Input: part model. Units: mm. Frame: model coordinates. A direction names the side the tool comes from. Give positions to 0.01 mm unless a question says otherwise; leave off trailing zeros. Loops run counter-clockwise (first coordinate to the right, second up) from the corner with the lowest first, then second, coordinate; pieces in that order, holes last. Notation, with made-up numbers: (-20, -5) -> (34, -5) arc R10 ccw to (34, 9) -> close; hole circle Ø7 at (-4.5, 84.25). An arc over 180 degrees is marked (long way). Answer as a JSON object with one key per item and string values.
```python
from build123d import *

# Parameters (mm, degrees)
BOSS_EXTRUDE2_OUTLINE_R   = 1.35
BOSS_EXTRUDE2_OUTLINE_W   = 11
BOSS_EXTRUDE2_OUTLINE_H   = 69
BOSS_EXTRUDE2_OUTLINE_R_2 = 12.095
BOSS_EXTRUDE2_OUTLINE_R_3 = 1.143
BOSS_EXTRUDE2_DEPTH       = 3.175
CUT_EXTRUDE1_DEPTH        = 6.35
FILLET1_R                 = 0.5


# Read off the part's stored shape, not the designer's step: Boss-Extrude2
with BuildPart() as part:
    # Boss-Extrude2 outline → Boss-Extrude2 (new body)
    with BuildSketch(Plane(origin=(0, 0, 0), x_dir=(1, 0, 0), z_dir=(0, 1, 0))):
        with BuildLine():
            ThreePointArc((-13.319120077, -43.925216134), (-10.126305957, -47.701325441), (-5.276948898, -48.669209533))
            ThreePointArc((-5.276948898, -48.669209533), (0, -48.302004425), (5.276948898, -48.669209533))
            ThreePointArc((5.276948898, -48.669209533), (10.126305957, -47.701325441), (13.319120077, -43.925216134))
            Line((13.319120077, -43.925216134), (17.904063474, -31.950549264))
            Line((17.904063474, -31.950549264), (23.040433069, -33.917198033))
            Line((23.040433069, -33.917198033), (18.455489673, -45.891864903))
            ThreePointArc((18.455489673, -45.891864903), (18.309924074, -50.834725832), (21.272807595, -54.79381471))
            ThreePointArc((21.272807595, -54.79381471), (26.466137741, -58.99482374), (30.845959646, -64.038266509))
            ThreePointArc((30.845959646, -64.038266509), (30.722917613, -61.793165345), (29.939937248, -59.685427143))
            Line((29.939937248, -59.685427143), (23.761921217, -48.539993511))
            Line((23.761921217, -48.539993511), (28.572329606, -45.873540599))
            Line((28.572329606, -45.873540599), (34.750345491, -57.018976288))
            ThreePointArc((34.750345491, -57.018976288), (39.797694407, -60.728851606), (45.899993549, -59.314337155))
            ThreePointArc((45.899993549, -59.314337155), (49.682691748, -56.183895741), (53.252452412, -52.812652955))
            ThreePointArc((53.252452412, -52.812652955), (55.400241506, -46.895968251), (52.284336639, -41.426846498))
            Line((52.284336639, -41.426846498), (41.919203487, -33.87844485))
            Line((41.919203487, -33.87844485), (45.152040904, -29.428864843))
            Line((45.152040904, -29.428864843), (55.532494673, -36.970706015))
            ThreePointArc((55.532494673, -36.970706015), (61.693781059, -38.244294688), (66.657056834, -34.377852961))
            ThreePointArc((66.657056834, -34.377852961), (74.442262703, 9.129596032), (56.374397975, 49.466425512))
            ThreePointArc((56.374397975, 49.466425512), (50.654117331, 52.01932544), (44.991624855, 49.340690033))
            Line((44.991624855, 49.340690033), (36.78429665, 39.55957716))
            Line((36.78429665, 39.55957716), (32.571052213, 43.094909013))
            Line((32.571052213, 43.094909013), (40.778380417, 52.876021886))
            ThreePointArc((40.778380417, 52.876021886), (42.433039833, 58.917628535), (38.925607882, 64.107698843))
            ThreePointArc((38.925607882, 64.107698843), (0, 75), (-38.925607882, 64.107698843))
            ThreePointArc((-38.925607882, 64.107698843), (-42.433039833, 58.917628535), (-40.778380417, 52.876021886))
            Line((-40.778380417, 52.876021886), (-32.571052213, 43.094909013))
            Line((-32.571052213, 43.094909013), (-36.78429665, 39.55957716))
            Line((-36.78429665, 39.55957716), (-44.991624855, 49.340690033))
            ThreePointArc((-44.991624855, 49.340690033), (-50.654117331, 52.01932544), (-56.374397975, 49.466425512))
            ThreePointArc((-56.374397975, 49.466425512), (-74.442262703, 9.129596032), (-66.657056834, -34.377852961))
            ThreePointArc((-66.657056834, -34.377852961), (-61.693781059, -38.244294688), (-55.532494673, -36.970706015))
            Line((-55.532494673, -36.970706015), (-45.152040904, -29.428864843))
            Line((-45.152040904, -29.428864843), (-41.919203487, -33.87844485))
            Line((-41.919203487, -33.87844485), (-52.284336639, -41.426846498))
            ThreePointArc((-52.284336639, -41.426846498), (-55.400241506, -46.895968251), (-53.252452412, -52.812652955))
            ThreePointArc((-53.252452412, -52.812652955), (-49.682691748, -56.183895741), (-45.899993549, -59.314337155))
            ThreePointArc((-45.899993549, -59.314337155), (-39.797694407, -60.728851606), (-34.750345491, -57.018976288))
            Line((-34.750345491, -57.018976288), (-28.572329606, -45.873540599))
            Line((-28.572329606, -45.873540599), (-23.761921217, -48.539993511))
            Line((-23.761921217, -48.539993511), (-29.939937248, -59.685427143))
            ThreePointArc((-29.939937248, -59.685427143), (-30.722917613, -61.793165345), (-30.845959646, -64.038266509))
            ThreePointArc((-30.845959646, -64.038266509), (-26.466137741, -58.99482374), (-21.272807595, -54.79381471))
            ThreePointArc((-21.272807595, -54.79381471), (-18.309924074, -50.834725832), (-18.455489673, -45.891864903))
            Line((-18.455489673, -45.891864903), (-23.040433069, -33.917198033))
            Line((-23.040433069, -33.917198033), (-17.904063474, -31.950549264))
            Line((-17.904063474, -31.950549264), (-13.319120077, -43.925216134))
        make_face()
        with Locations((-43.735655662, -41.075447944)):
            Circle(BOSS_EXTRUDE2_OUTLINE_R, mode=Mode.SUBTRACT)
        with Locations((-38.234289702, -39.23697625)):
            Circle(BOSS_EXTRUDE2_OUTLINE_R, mode=Mode.SUBTRACT)
        with Locations((-6.55476095, -38.026099982)):
            Circle(BOSS_EXTRUDE2_OUTLINE_R, mode=Mode.SUBTRACT)
        with Locations((-44.385223141, -22.074211772)):
            Circle(BOSS_EXTRUDE2_OUTLINE_R, mode=Mode.SUBTRACT)
        with Locations((-58.910067426, 0.102907352)):
            Rectangle(BOSS_EXTRUDE2_OUTLINE_W, BOSS_EXTRUDE2_OUTLINE_H, mode=Mode.SUBTRACT)
        with Locations((-42.910067426, -11.1)):
            Circle(BOSS_EXTRUDE2_OUTLINE_R, mode=Mode.SUBTRACT)
        with Locations((-26.905821676, -20.904643604)):
            Circle(BOSS_EXTRUDE2_OUTLINE_R_2, mode=Mode.SUBTRACT)
        with Locations((-11.160067426, -11.1)):
            Circle(BOSS_EXTRUDE2_OUTLINE_R, mode=Mode.SUBTRACT)
        with Locations((38.234289702, -39.23697625)):
            Circle(BOSS_EXTRUDE2_OUTLINE_R, mode=Mode.SUBTRACT)
        with Locations((43.735655662, -41.075447944)):
            Circle(BOSS_EXTRUDE2_OUTLINE_R, mode=Mode.SUBTRACT)
        with Locations((0, -25.409190322)):
            Circle(BOSS_EXTRUDE2_OUTLINE_R_2, mode=Mode.SUBTRACT)
        with Locations((10.597026674, -15.930038136)):
            Circle(BOSS_EXTRUDE2_OUTLINE_R, mode=Mode.SUBTRACT)
        with Locations((26.905821676, -20.904643604)):
            Circle(BOSS_EXTRUDE2_OUTLINE_R_2, mode=Mode.SUBTRACT)
        with Locations((11.160067426, -11.1)):
            Circle(BOSS_EXTRUDE2_OUTLINE_R, mode=Mode.SUBTRACT)
        with Locations((41.601681906, -17.457756634)):
            Circle(BOSS_EXTRUDE2_OUTLINE_R, mode=Mode.SUBTRACT)
        with Locations((42.910067426, -11.1)):
            Circle(BOSS_EXTRUDE2_OUTLINE_R, mode=Mode.SUBTRACT)
        with Locations((58.910067426, 0.102907352)):
            Rectangle(BOSS_EXTRUDE2_OUTLINE_W, BOSS_EXTRUDE2_OUTLINE_H, mode=Mode.SUBTRACT)
        with Locations((-42.910067426, 11.1)):
            Circle(BOSS_EXTRUDE2_OUTLINE_R, mode=Mode.SUBTRACT)
        with Locations((-42.910067426, 18.234848025)):
            Circle(BOSS_EXTRUDE2_OUTLINE_R, mode=Mode.SUBTRACT)
        with Locations((-45.13872464, 31.997163897)):
            Circle(BOSS_EXTRUDE2_OUTLINE_R, mode=Mode.SUBTRACT)
        with Locations((-11.160067426, 11.1)):
            Circle(BOSS_EXTRUDE2_OUTLINE_R, mode=Mode.SUBTRACT)
        with Locations((-29.939937248, 24.651901309)):
            Circle(BOSS_EXTRUDE2_OUTLINE_R_2, mode=Mode.SUBTRACT)
        with Locations((-13.346873881, 34.693819966)):
            Circle(BOSS_EXTRUDE2_OUTLINE_R, mode=Mode.SUBTRACT)
        with Locations((-43.735655662, 41.075447944)):
            Circle(BOSS_EXTRUDE2_OUTLINE_R, mode=Mode.SUBTRACT)
        with Locations((-33.21799214, 49)):
            Circle(BOSS_EXTRUDE2_OUTLINE_R, mode=Mode.SUBTRACT)
        with Locations((-19, 49)):
            Circle(BOSS_EXTRUDE2_OUTLINE_R_2, mode=Mode.SUBTRACT)
        with Locations((-4.78200786, 49)):
            Circle(BOSS_EXTRUDE2_OUTLINE_R, mode=Mode.SUBTRACT)
        with Locations((-6.731, 61.422565207)):
            Circle(BOSS_EXTRUDE2_OUTLINE_R_3, mode=Mode.SUBTRACT)
        with Locations((11.160067426, 11.1)):
            Circle(BOSS_EXTRUDE2_OUTLINE_R, mode=Mode.SUBTRACT)
        with Locations((0, 29.793589551)):
            Circle(BOSS_EXTRUDE2_OUTLINE_R_2, mode=Mode.SUBTRACT)
        with Locations((13.346873881, 34.693819966)):
            Circle(BOSS_EXTRUDE2_OUTLINE_R, mode=Mode.SUBTRACT)
        with Locations((29.939937248, 24.651901309)):
            Circle(BOSS_EXTRUDE2_OUTLINE_R_2, mode=Mode.SUBTRACT)
        with Locations((42.910067426, 11.1)):
            Circle(BOSS_EXTRUDE2_OUTLINE_R, mode=Mode.SUBTRACT)
        with Locations((42.910067426, 18.234848025)):
            Circle(BOSS_EXTRUDE2_OUTLINE_R, mode=Mode.SUBTRACT)
        with Locations((45.13872464, 31.997163897)):
            Circle(BOSS_EXTRUDE2_OUTLINE_R, mode=Mode.SUBTRACT)
        with Locations((4.78200786, 49)):
            Circle(BOSS_EXTRUDE2_OUTLINE_R, mode=Mode.SUBTRACT)
        with Locations((19, 49)):
            Circle(BOSS_EXTRUDE2_OUTLINE_R_2, mode=Mode.SUBTRACT)
        with Locations((33.21799214, 49)):
            Circle(BOSS_EXTRUDE2_OUTLINE_R, mode=Mode.SUBTRACT)
        with Locations((6.731, 61.422565207)):
            Circle(BOSS_EXTRUDE2_OUTLINE_R_3, mode=Mode.SUBTRACT)
        with Locations((43.735655662, 41.075447944)):
            Circle(BOSS_EXTRUDE2_OUTLINE_R, mode=Mode.SUBTRACT)
    extrude(amount=BOSS_EXTRUDE2_DEPTH)

    # Sketch3 → Cut-Extrude1 (cut)
    with BuildSketch(Plane(origin=(0, 3.175, 0), x_dir=(1, 0, 0), z_dir=(0, 1, 0))):
        with BuildLine():
            Line((-30.581569801, 39.557143331), (-34.365473638, 44.066624323))
            ThreePointArc((-34.365473638, 44.066624323), (-35.920574868, 42.808474147), (-37.42965141, 41.495473884))
            Line((-37.42965141, 41.495473884), (-33.645747573, 36.985992892))
            ThreePointArc((-33.645747573, 36.985992892), (-32.139380484, 38.302222156), (-30.581569801, 39.557143331))
        make_face()
        with BuildLine():
            Line((-41.563047759, -27.79411918), (-46.321630401, -31.259553973))
            ThreePointArc((-46.321630401, -31.259553973), (-45.173194515, -32.897350272), (-43.966878649, -34.492995513))
            Line((-43.966878649, -34.492995513), (-39.208296007, -31.02756072))
            ThreePointArc((-39.208296007, -31.02756072), (-40.418019242, -29.434396894), (-41.563047759, -27.79411918))
        make_face()
        with BuildLine():
            Line((-22.47184145, -44.665605804), (-25.325774778, -49.814237819))
            ThreePointArc((-25.325774778, -49.814237819), (-27.09237079, -48.875930708), (-28.824253607, -47.874999338))
            Line((-28.824253607, -47.874999338), (-25.970320279, -42.726367323))
            ThreePointArc((-25.970320279, -42.726367323), (-24.240481012, -43.730985357), (-22.47184145, -44.665605804))
        make_face()
        with BuildLine():
            Line((25.970320279, -42.726367323), (28.824253607, -47.874999338))
            ThreePointArc((28.824253607, -47.874999338), (27.09237079, -48.875930708), (25.325774778, -49.814237819))
            Line((25.325774778, -49.814237819), (22.47184145, -44.665605804))
            ThreePointArc((22.47184145, -44.665605804), (24.240481012, -43.730985357), (25.970320279, -42.726367323))
        make_face()
        with BuildLine():
            Line((39.208296007, -31.02756072), (43.966878649, -34.492995513))
            ThreePointArc((43.966878649, -34.492995513), (45.173194515, -32.897350272), (46.321630401, -31.259553973))
            Line((46.321630401, -31.259553973), (41.563047759, -27.79411918))
            ThreePointArc((41.563047759, -27.79411918), (40.418019242, -29.434396894), (39.208296007, -31.02756072))
        make_face()
        with BuildLine():
            Line((33.645747573, 36.985992892), (37.42965141, 41.495473884))
            ThreePointArc((37.42965141, 41.495473884), (35.920574868, 42.808474147), (34.365473638, 44.066624323))
            Line((34.365473638, 44.066624323), (30.581569801, 39.557143331))
            ThreePointArc((30.581569801, 39.557143331), (32.139380484, 38.302222156), (33.645747573, 36.985992892))
        make_face()
    extrude(amount=-CUT_EXTRUDE1_DEPTH, mode=Mode.SUBTRACT)

    # Fillet1
    fillet1_edges = [part.edges().sort_by_distance(p)[0] for p in [
        (-30.845959646, 1.5875, 64.038266509),
        (30.845959646, 1.5875, 64.038266509),
    ]]
    fillet(fillet1_edges, radius=FILLET1_R)


solid = part.part
```
Q1. Section B-B, the plane x = -61. Return the cut outline in (y, z) (3 decimals), then the cut area to 3 significant figures.
Evaluation:
{"outline": "(0, -43.635) -> (3.175, -43.635) -> (3.175, -34.603) -> (0, -34.603) -> close; (0, 34.397) -> (3.175, 34.397) -> (3.175, 38.372) -> (0, 38.372) -> close", "area": "41.3 mm2"}
Q2. Access query for faces 1 (the cylindrical face through (50.74, 1.57, -52.02)), 2 (the flat face through (64.41, 2, 0)). Directions: +Z, -Z, +X, -X, +Y, -Y. A direction counts if a zero-diameter tool reaches every point of the face in a straight line with its end or side. Return the directions, or none.
Evaluation:
{"face 1": "-Z, +Y, -Y", "face 2": "+Y, -Y"}
Q3. Pin query (flat end, axial travel): pin 1 (19.5 mm diameter, centred on x = 0, z = -29.79, fed in from +Y). Return the tip coordinate at first contact, or that it passes through.
Evaluation:
{"pin 1": "passes through"}
Q4. Section A-A, the plane x = 0. Return the cut outline in (y, z) (3 decimals), then the cut area to 3 significant figures.
Evaluation:
{"outline": "(0, -75) -> (3.175, -75) -> (3.175, -41.889) -> (0, -41.889) -> close; (0, -17.699) -> (3.175, -17.699) -> (3.175, 13.314) -> (0, 13.314) -> close; (0, 37.504) -> (3.175, 37.504) -> (3.175, 48.302) -> (0, 48.302) -> close", "area": "238 mm2"}
Q5. Draft query along Z for faces 3 (the cylindrical face through (-39.886, 1.565, 60.747)), 4 (the flat face through (26.93, 1.61, 44.46)), 5 (the cylindrical face through (-74.363, 1.565, -9.753)). Return one class per face: +Z half, -Z half, draft (parallel to the pull), parting line (faces both ways), or undercut.
Evaluation:
{"face 3": "+Z half", "face 4": "undercut", "face 5": "parting line"}
Q6. Ray query, line 1 along X through (y, z) = (0.15, -4); line 2 along Z through (x, y) = (9, 2.9); line 3 along Z through (x, y) = (30, 1.55). Return the intervals inside material, ascending.
Evaluation:
{"line 1": "x = -74.89 to -64.41, -53.41 to 53.41, 64.41 to 74.89", "line 2": "z = -74.46 to -55.8, -42.2 to -37.87, -21.71 to 17.33, 33.49 to 48.24", "line 3": "z = -68.74 to -54.03, -43.97 to -36.75, -12.56 to 9.21, 32.6 to 48.45, 59.8 to 62.9"}
Q7. Section C-C, the plane y = 0.85. Give the number of separate pieces and of enclosed holes in the cut face, then the cut area to 3 significant figures.
Evaluation:
{"separate pieces": "1", "enclosed holes": "40", "area": "9,870 mm2"}
